For this review, take the finished solid that the model builds, in its own axes (mm). A direction names the side the tool comes from. Round coordinates to 2 decimals unless told otherwise and drop trailing zeros. Write each loop counter-clockwise with the first axis right and the second up, starting at its lowest first coordinate (ties: lowest second). Pieces come first, ordered by that corner, then holes. Notation, with made-up numbers: (20, 38.25) - (59, 38.25) arc R22 ccw to (59, 47.25) - close; hole circle Ø6 at (-10.5, 62). An arc over 180 degrees is marked (long way). One line per item, written item: value. Start each with the question number.
Q1. Tool access review of faces 5 (the face through (12, 66.275, -56)), 6 (the face through (0, 6, -54)): name each direction out of +Z, -Z, +X, -X, +Y, -Y from which nothing blocks a thin tool from reaching the whole face with its end or side.
Q2. Add section A-A on z = -20. Write out the cut boundary in (x, y), and give its area (3 significant figures).
Q3. Clearance check with flat-ended pins moving along their axes: pin 1 Ø7.5 at (x, z) = (11, -70.5) entering from -Y; pin 2 Ø4 at (x, y) = (2.5, 39.5) entering from -Z; pin 3 Ø12 at (y, z) = (10.5, -69.5) entering from -X; pin 4 Ø8 at (x, z) = (20, -115.5) entering from -Y. State where each tip first meets the part, or that it passes through.
Q4. Add section C-C on x = 21.5. Write out the cut boundary in (y, z).
Q5. Mouldability with a two-part tool opening along Z and no side actions: class faces 1 (the face through (12.325, 10.414, -57.447)), 2 (the face through (12, 2, 10)), 3 (the face through (12.325, 0.225, -63.95)), 4 (the face through (25, 6, -54)) as +Z half, -Z half, draft (parallel to the pull), parting line (faces both ways), or undercut.
Q6. Add section B-B on y = 42.5. Write out the cut boundary in (x, z), and give its area (3 significant figures).
Q7. For probe 1 along Z at (x, y) = (1.5, -30); probe 2 along Y at (x, z) = (10, -74.5); probe 3 along Y at (x, z) = (20, -5), list the stretches that pass through material, from the lowest coordinate up.
```python
from build123d import *

# Parameters (mm, degrees)
F1_DEPTH = 25


with BuildPart() as f1:
    # F0 (on Right) → F1 (new body)
    with BuildSketch(Plane.YZ):
        Polygon((-57.0327825844, 10), (-73.7252708524, 10), (-63.7252708524, 0), (-47.0327825844, 0), align=None)
        Polygon((76.2747291476, 10), (-57.0327825844, 10), (-47.0327825844, 0), (66.2747291476, 0), (76.2747291476, 0), align=None)
        Polygon((76.2747291476, -123.307511732), (76.2747291476, 0), (66.2747291476, 0), (66.2747291476, -113.307511732), align=None)
        Polygon((66.2747291476, -113.307511732), (66.2747291476, -130), (76.2747291476, -140), (76.2747291476, -123.307511732), align=None)
        Polygon((-47.0327825844, 0), (-63.7252708524, 0), (66.2747291476, -130), (66.2747291476, -113.307511732), align=None)
    extrude(amount=F1_DEPTH)


solid = f1.part
```
Result set:
1. face 5: +X, -X
1. face 6: +Z, -Z, -X, +Y, -Y
2. outline: (0, -43.73) - (25, -43.73) - (25, -27.03) - (0, -27.03) - close; (0, 66.27) - (25, 66.27) - (25, 76.27) - (0, 76.27) - close
2. area: 667 mm^2
3. pin 1: stops at y = 3.02
3. pin 2: stops at z = -105.23
3. pin 3: stops at x = 0
3. pin 4: stops at y = 47.77
4. outline: (-73.73, 10) - (76.27, -140) - (76.27, 10) - close; hole (-47.03, 0) - (66.27, -113.31) - (66.27, 0) - close
5. face 1: undercut
5. face 2: +Z half
5. face 3: -Z half
5. face 4: draft
6. outline: (0, -106.23) - (25, -106.23) - (25, -89.53) - (0, -89.53) - close; (0, 0) - (25, 0) - (25, 10) - (0, 10) - close
6. area: 667 mm^2
7. probe 1: z = -33.73 to -17.03, 0 to 10
7. probe 2: y = 10.77 to 27.47, 66.27 to 76.27
7. probe 3: y = -58.73 to -42.03, 66.27 to 76.27
